```python
from build123d import *

# Parameters (mm, degrees)
F1_DEPTH = 12.7
F2_R     = 29.530414
F3_DEPTH = 152.4
F4_R     = 29.530414
F5_DEPTH = 12.7


with BuildPart() as f1:
    # F0 (on Front) → F1 (new body)
    with BuildSketch(Plane.XZ):
        Polygon((11.869742, 40.42463), (-11.869742, 40.42463), (-31.840668, 27.590096), (-41.702406, 5.995901), (-38.323925, -17.50195), (-22.777869, -35.443056), (0, -42.131241), (22.777869, -35.443056), (38.323925, -17.50195), (41.702406, 5.995901), (31.840668, 27.590096), align=None)
    extrude(amount=F1_DEPTH)

    # F2 (on face) → F3 (join)
    with BuildSketch(Plane(origin=(0, 0, 0), x_dir=(-1, 0, 0), z_dir=(0, 1, 0))):
        Circle(F2_R)
    extrude(amount=F3_DEPTH)

    # F4 (on face) → F5 (join)
    with BuildSketch(Plane(origin=(0, 152.4, 0), x_dir=(-1, 0, 0), z_dir=(0, 1, 0))):
        Polygon((45.335108, 23.784663), (2.069431, 51.153686), (-43.265676, 27.369023), (-45.335108, -23.784663), (-2.069431, -51.153686), (43.265676, -27.369023), align=None)
        Circle(F4_R, mode=Mode.SUBTRACT)
    extrude(amount=-F5_DEPTH)


solid = f1.part
```
Check sheet for the modelled part. Datum: model origin and axes. Units: mm. A direction names the side the tool comes from. Round coordinates to 2 decimals unless told otherwise and drop trailing zeros. Order: outer loops, then holes, each group sorted by start corner. A loop starts at its lowest first (then second) coordinate and runs counter-clockwise, first axis right, second up. Notation, with made-up numbers: (15, 42.25) -> (71, 42.25) arc R7 cw to (71, 49.25) -> close; hole circle Ø6 at (89.25, 16). An arc over 180 degrees is marked (long way). Use CSV: the item, a comma, the result in double quotes.
(1) Material ranges on line 1 along Y through (x, z) = (-16.5, 28); line 2 along X through (y, z) = (65.5, -0.5); line 3 along Y through (x, z) = (31.5, 32), recorded low to high. Write a range as from..to.
Worked out:
line 1,"-12.7..0, 139.7..152.4"
line 2,"-29.53..29.53"
line 3,"139.7..152.4"
(2) Cross-section at A-A (x = -35). Record the boundary of the cut face in (y, z), and give its area (3 significant figures).
Worked out:
outline,"(-12.7, -21.34) -> (0, -21.34) -> (0, 20.67) -> (-12.7, 20.67) -> close; (139.7, -31.71) -> (152.4, -31.71) -> (152.4, 30.32) -> (139.7, 30.32) -> close"
area,"1,320 mm²"
(3) Depth check by flat-ended pin: pin 1 (6 mm diameter, centred on x = 3.5, y = 93, fed in from +Z); pin 2 (2 mm diameter, centred on x = -16.5, y = 126, fed in from +Z); pin 3 (12 mm diameter, centred on x = -0.5, y = 90.5, fed in from -Z). Enter the tip coordinate at first touch or a pass-through.
Worked out:
pin 1,"z = 29.53"
pin 2,"z = 25.14"
pin 3,"z = -29.53"
(4) Draft check along Y on faces 1 (the face through (-9.5, 0, -28.2)), 2 (the face through (1, 152.4, 1)), 3 (the face through (-44.286, 146.139, -2.15)). Enter one of: pulls with the +Y half, pulls with the -Y half, needs draft (parallel to the pull), parting line crosses it, or undercut.
Worked out:
face 1,"undercut"
face 2,"pulls with the +Y half"
face 3,"needs draft"
(5) Cross-section at B-B (z = -8.5). Record the boundary of the cut face in (x, y).
Worked out:
outline,"(-44.03, 139.7) -> (-28.28, 139.7) -> (-28.28, 0) -> (-39.62, 0) -> (-39.62, -12.7) -> (39.62, -12.7) -> (39.62, 0) -> (28.28, 0) -> (28.28, 139.7) -> (44.72, 139.7) -> (44.72, 152.4) -> (-44.03, 152.4) -> close"
(6) Cross-section at D-D (x = -5). Record the boundary of the cut face in (y, z), and give its area (3 significant figures).
Worked out:
outline,"(-12.7, -40.66) -> (0, -40.66) -> (0, -29.1) -> (139.7, -29.1) -> (139.7, -47.44) -> (152.4, -47.44) -> (152.4, 49.3) -> (139.7, 49.3) -> (139.7, 29.1) -> (0, 29.1) -> (0, 40.42) -> (-12.7, 40.42) -> close"
area,"10,400 mm²"
(7) Cross-section at C-C (y = 82). Record the boundary of the cut face in (x, z).
Worked out:
outline,"circle Ø59.06 at (0, 0)"
(8) Tool access check on faces 4 (the face through (21.995, -6.261, 33.918)), 5 (the face through (-40.037, -6.261, -5.589)), 6 (the face through (-36.703, -6.261, 16.944)). Record the directions out of +Z, -Z, +X, -X, +Y, -Y that give a thin tool (end or side, any length) a straight path to the whole face; none if there is none.
Worked out:
face 4,"+Z, +X, -Y"
face 5,"-Z, -X, -Y"
face 6,"+Z, -X, -Y"
